```python
from build123d import *

# Parameters (mm, degrees)
SKETCH1_R           = 3.5
BOSS_EXTRUDE1_DEPTH = 30
SKETCH3_R           = 1.75
BOSS_EXTRUDE2_DEPTH = 1


with BuildPart() as part:
    # Sketch1 → Boss-Extrude1 (new body)
    with BuildSketch(Plane.XY):
        Circle(SKETCH1_R)
    extrude(amount=BOSS_EXTRUDE1_DEPTH)

    # Sketch3 → Boss-Extrude2 (add)
    with BuildSketch(Plane.XY.offset(30)):
        with BuildLine():
            Line((0, 10.5), (-3.299831646, 1.166666667))
            ThreePointArc((-3.299831646, 1.166666667), (0, -3.5), (3.299831646, 1.166666667))
            Line((3.299831646, 1.166666667), (0, 10.5))
        make_face()
        Circle(SKETCH3_R, mode=Mode.SUBTRACT)
    extrude(amount=BOSS_EXTRUDE2_DEPTH)


solid = part.part
```
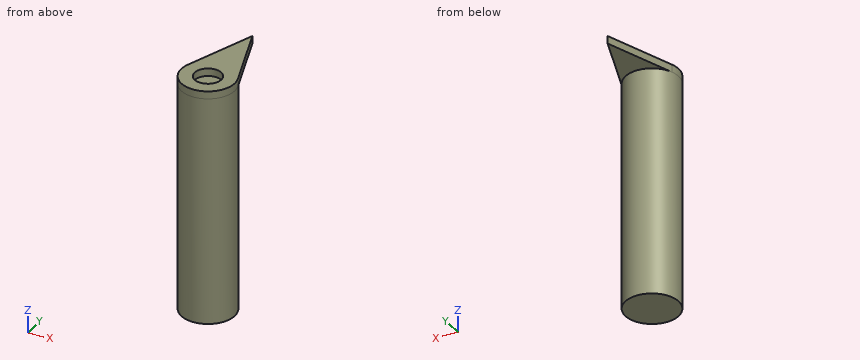
Verification items for the finished model (mm, model axes). Give positions to 0.01 mm unless a question says otherwise; leave off trailing zeros. Order: outer loops, then holes, each group sorted by start corner. A loop starts at its lowest first (then second) coordinate and runs counter-clockwise, first axis right, second up. Notation, with made-up numbers: M -12,-0.5 L 34,-0.5 A22 cw 34,22.5 Z; hole C 9.25,40 d2. An arc over 180 degrees is marked long. Answer in a Markdown table with one row per item. Add a question column.
Item 1: Gauge pin test, flat ends, axial feed: pin 1 (8 mm diameter, centred on y = 7, z = 11.5, fed in from +X); pin 2 (2 mm diameter, centred on y = -2, z = 13, fed in from +X); pin 3 (1.5 mm diameter, centred on x = -2, z = 24, fed in from +Y). Record the tip position at first contact, or that the pin passes through.
Item 2: Section check A-A, the plane y = 0. Enter the section's corners in (x, z), and give its area (4 significant figures).
Item 3: Section check C-C, the plane z = 3.5. Enter the section's corners in (x, y), and give its area (3 significant figures).
Item 4: Section check D-D, the plane y = 2.75. Enter the section's corners in (x, z).
Item 5: Scan lines: probe 1 along Y at (x, z) = (0, 25); probe 2 along Z at (x, y) = (-0.25, 4); probe 3 along Y at (x, z) = (-2.75, 28). Record each from-to range of solid material in increasing order. Write a range as from..to.
Item 6: Section check B-B, the plane x = -2.5. Enter the section's corners in (y, z), and give its area (3 significant figures).
Filled sheet:
| question | item | result |
|---|---|---|
| 1 | pin 1 | stops at x = 1.8 |
| 1 | pin 2 | stops at x = 3.35 |
| 1 | pin 3 | stops at y = 3.27 |
| 2 | outline | M -3.5,0 L 3.5,0 L 3.5,31 L 1.75,31 L 1.75,30 L -1.75,30 L -1.75,31 L -3.5,31 Z |
| 2 | area | 213.5 mm^2 |
| 3 | outline | C 0,0 d7 |
| 3 | area | 38.5 mm^2 |
| 4 | outline | M -2.74,30 L -2.17,30 L -2.17,0 L 2.17,0 L 2.17,30 L 2.74,30 L 2.74,31 L -2.74,31 Z |
| 5 | probe 1 | y = -3.5..3.5 |
| 5 | probe 2 | z = 30..31 |
| 5 | probe 3 | y = -2.17..2.17 |
| 6 | outline | M -2.45,0 L 2.45,0 L 2.45,30 L 3.43,30 L 3.43,31 L -2.45,31 Z |
| 6 | area | 153 mm^2 |
